Input: part model. Units: mm. Frame: model coordinates. A direction names the side the tool comes from. Round coordinates to 2 decimals unless told otherwise and drop trailing zeros. Loops run counter-clockwise (first coordinate to the right, second up) from the corner with the lowest first, then second, coordinate; pieces in that order, holes last. Notation, with made-up numbers: (-13.75, -18.75) -> (2.25, -18.75) arc R18 cw to (2.25, 10.25) -> close; hole circle Ø9 at (42, -4.75). An arc over 180 degrees is marked (long way). Answer as a JSON object with one key per item and string values. Group by question number.
Item 1: Material intervals for line 1 (X direction, y = 4, z = 0); line 2 (Z direction, x = 1.5, y = 4); line 3 (X direction, y = 8.5, z = -1.5), sorted ascending. Write a range as [from, to].
Item 2: Set-up query: faces 1 (the cylindrical face through (0.2, 6.9, 0.62)), 2 (the flat face through (4, 0, -2)). Return all of +Z, -Z, +X, -X, +Y, -Y with unobstructed straight access to the full face (end or side cutting, diameter ignored); none if empty.
Item 3: Section query C-C on y = 10.75. Return loops of the section in (x, z).
Item 4: Draft query along Z for faces 3 (the flat face through (0, 15, 0)), 4 (the cylindrical face through (-0.632, 4.437, 1.524)). Return one class per face: released by +Z, released by -Z, zero draft, split by the parting line, or undercut.
Item 5: Section query A-A on y = 2. Return loops of the section in (x, z).
Item 6: Pin query (flat end, axial travel): pin 1 (3 mm diameter, centred on y = 3, z = 4, fed in from -X); pin 2 (5 mm diameter, centred on y = 5, z = 2.5, fed in from +X); pin 3 (5 mm diameter, centred on x = 3.5, y = 2.5, fed in from +Z). Return the tip coordinate at first contact, or that it passes through.
Item 7: Section query B-B on y = 7. Return loops of the section in (x, z), and give its area (3 significant figures).
from build123d import *

# Parameters (mm, degrees)
SKETCH2_R           = 1.65
SKETCH2_R_2         = 0.65
BOSS_EXTRUDE1_DEPTH = 14
FILLET1_R           = 1


with BuildPart() as part:
    # Sketch2 → Boss-Extrude1 (new body)
    with BuildSketch(Plane(origin=(0, 0, 0), x_dir=(1, 0, 0), z_dir=(0, 1, 0))):
        with Locations(Location((0, 0, 0), (0, 0, 270))):
            Circle(SKETCH2_R)
        with Locations(Location((0, 0, 0), (0, 0, 270))):
            Circle(SKETCH2_R_2, mode=Mode.SUBTRACT)
    extrude(amount=BOSS_EXTRUDE1_DEPTH)

    # Sketch4 → Revolve1 (revolve)
    with BuildSketch(Plane.XY, mode=Mode.PRIVATE) as revolve1_sk:
        Polygon((2, 14), (4, 0), (5.010152545, 0), (3.010152545, 14), align=None)
        Polygon((2.867295402, 15), (3.010152545, 14), (0, 14), (0, 15), align=None)
    revolve(revolve1_sk.sketch.rotate(Axis((0, 0, 0), (0, 1, 0)), 90), axis=Axis((0, 0, 0), (0, 1, 0)))

    # Chamfer1: read off the stored shape, not the designer's step
    # Chamfer1 outline → Chamfer1 (revolve)
    with BuildSketch(Plane.XY):
        Polygon((1.65, 9), (2.58125, 9.93125), (2.58125, 14), (1.65, 14), align=None)
    revolve(axis=Axis((0, 0, 0), (0, 1, 0)))

    # Fillet1
    fillet1_edges = [part.edges().sort_by_distance(p)[0] for p in [
        (0, 15, 2.867295402),
    ]]
    fillet(fillet1_edges, radius=FILLET1_R)


solid = part.part
Solved:
{
 "1": {"line 1": "[-4.44, -3.43], [-1.65, -0.65], [0.65, 1.65], [3.43, 4.44]", "line 2": "[-4.18, -3.08], [-0.69, 0.69], [3.08, 4.18]", "line 3": "[-3.49, -2.35], [-0.69, 0.69], [2.35, 3.49]"},
 "2": {"face 1": "-Y", "face 2": "+Z, -Z, +X, -X, -Y"},
 "3": {"outline": "circle Ø6.95 at (0, 0); hole circle Ø1.3 at (0, 0)"},
 "4": {"face 3": "zero draft", "face 4": "undercut"},
 "5": {"outline": "circle Ø9.45 at (0, 0); circle Ø3.3 at (0, 0); hole circle Ø7.43 at (0, 0); hole circle Ø1.3 at (0, 0)"},
 "6": {"pin 1": "x = -3.87", "pin 2": "x = 4.49", "pin 3": "z = 4.64"},
 "7": {"outline": "circle Ø8.02 at (0, 0); circle Ø3.3 at (0, 0); hole circle Ø6 at (0, 0); hole circle Ø1.3 at (0, 0)", "area": "29.5 mm²"}
}
